```python
from build123d import *

# Parameters (mm, degrees)
BOSS_EXTRUDE1_DEPTH     = 35
SKETCH2_R               = 1.5
CUT_EXTRUDE1_DEPTH      = 31
CUT_EXTRUDE1_DEPTH_BACK = 31
SKETCH3_R               = 1.75
CUT_EXTRUDE2_DEPTH      = 6
FILLET1_R               = 4
FILLET2_R               = 2
CHAMFER1_SIZE           = 0.5


with BuildPart() as part:
    # Sketch1 → Boss-Extrude1 (new body)
    with BuildSketch(Plane.XY):
        with BuildLine():
            ThreePointArc((-10, -15.801582199), (-18.048902858, 4.891534078), (-0.652620588, 18.688608465))
            Line((-0.652620588, 18.688608465), (-0.792218575, 22.686171773))
            ThreePointArc((-0.792218575, 22.686171773), (-2.292863817, 22.583905232), (-3.783442178, 22.382483448))
            ThreePointArc((-3.783442178, 22.382483448), (-22.463854977, 3.265764775), (-10, -20.378665314))
            Line((-10, -20.378665314), (-10, -15.801582199))
        make_face()
        with BuildLine():
            Line((0, -22.7), (0, -18.7))
            ThreePointArc((0, -18.7), (-5.205785862, -17.960784882), (-10, -15.801582199))
            Line((-10, -15.801582199), (-10, -20.378665314))
            ThreePointArc((-10, -20.378665314), (-5.132947368, -22.112052173), (0, -22.7))
        make_face()
        with BuildLine():
            ThreePointArc((10, -15.801582199), (5.205785862, -17.960784882), (0, -18.7))
            Line((0, -18.7), (0, -22.7))
            ThreePointArc((0, -22.7), (5.132947368, -22.112052173), (10, -20.378665314))
            Line((10, -20.378665314), (10, -15.801582199))
        make_face()
        with BuildLine():
            Line((0.792218575, 22.686171773), (0.652620588, 18.688608465))
            ThreePointArc((0.652620588, 18.688608465), (18.048902858, 4.891534078), (10, -15.801582199))
            Line((10, -15.801582199), (10, -20.378665314))
            ThreePointArc((10, -20.378665314), (22.463854977, 3.265764775), (3.783442178, 22.382483448))
            ThreePointArc((3.783442178, 22.382483448), (2.292863817, 22.583905232), (0.792218575, 22.686171773))
        make_face()
        with BuildLine():
            ThreePointArc((10, -20.378665314), (5.132947368, -22.112052173), (0, -22.7))
            Line((0, -22.7), (0, -32))
            Line((0, -32), (30, -32))
            Line((30, -32), (30, -27))
            Line((30, -27), (16.621334686, -27))
            ThreePointArc((16.621334686, -27), (11.939344029, -25.060655971), (10, -20.378665314))
        make_face()
        with BuildLine():
            Line((0, -32), (0, -22.7))
            ThreePointArc((0, -22.7), (-5.132947368, -22.112052173), (-10, -20.378665314))
            ThreePointArc((-10, -20.378665314), (-11.939344029, -25.060655971), (-16.621334686, -27))
            Line((-16.621334686, -27), (-30, -27))
            Line((-30, -27), (-30, -32))
            Line((-30, -32), (0, -32))
        make_face()
        with BuildLine():
            ThreePointArc((-3.783442178, 22.382483448), (-2.292863817, 22.583905232), (-0.792218575, 22.686171773))
            Line((-0.792218575, 22.686171773), (-1.029566174, 29.482917727))
            Line((-1.029566174, 29.482917727), (-4.027738655, 29.378219237))
            Line((-4.027738655, 29.378219237), (-3.783442178, 22.382483448))
        make_face()
        with BuildLine():
            Line((1.029566174, 29.482917727), (0.792218575, 22.686171773))
            ThreePointArc((0.792218575, 22.686171773), (2.292863817, 22.583905232), (3.783442178, 22.382483448))
            Line((3.783442178, 22.382483448), (4.027738655, 29.378219237))
            Line((4.027738655, 29.378219237), (1.029566174, 29.482917727))
        make_face()
    extrude(amount=BOSS_EXTRUDE1_DEPTH)

    # Sketch2 → Cut-Extrude1 (cut, two sides)
    with BuildSketch(Plane(origin=(0, 0, 0), x_dir=(0, 0, -1), z_dir=(1, 0, 0))) as cut_extrude1_sk:
        with Locations((-30, 25.880351342)):
            Circle(SKETCH2_R)
        with Locations((-5, 25.880351342)):
            Circle(SKETCH2_R)
    extrude(amount=CUT_EXTRUDE1_DEPTH, mode=Mode.SUBTRACT)
    extrude(cut_extrude1_sk.sketch, amount=-CUT_EXTRUDE1_DEPTH_BACK, mode=Mode.SUBTRACT)

    # Sketch3 → Cut-Extrude2 (cut, through all)
    with BuildSketch(Plane(origin=(0, -27, 0), x_dir=(1, 0, 0), z_dir=(0, 1, 0))):
        with Locations((-25, -5)):
            Circle(SKETCH3_R)
        with Locations((-25, -30)):
            Circle(SKETCH3_R)
        with Locations((25, -30)):
            Circle(SKETCH3_R)
        with Locations((25, -5)):
            Circle(SKETCH3_R)
    extrude(amount=-CUT_EXTRUDE2_DEPTH, mode=Mode.SUBTRACT)

    # Fillet1
    fillet1_edges = [part.edges().sort_by_distance(p)[0] for p in [
        (-10, -20.378665314, 17.5),
        (10, -20.378665314, 17.5),
    ]]
    fillet(fillet1_edges, radius=FILLET1_R)

    # Fillet2
    fillet2_edges = [part.edges().sort_by_distance(p)[0] for p in [
        (-3.783442178, 22.382483448, 17.5),
        (-0.652620588, 18.688608465, 17.5),
        (0.652620588, 18.688608465, 17.5),
        (3.783442178, 22.382483448, 17.5),
    ]]
    fillet(fillet2_edges, radius=FILLET2_R)

    # Chamfer1
    chamfer1_edges = [part.edges().sort_by_distance(p)[0] for p in [
        (30, -29.5, 35),
        (-0.874302959, 25.03676097, 0),
        (-0.874302959, 25.03676097, 35),
        (-22.357902089, 3.926094008, 0),
        (-17.579381492, -6.376154512, 0),
        (0.874302959, 25.03676097, 0),
        (1.190855047, 19.229149784, 0),
        (-1.190855047, 19.229149784, 0),
        (-17.579381492, -6.376154512, 35),
        (0.874302959, 25.03676097, 35),
        (-22.357902089, 3.926094008, 35),
        (1.190855047, 19.229149784, 35),
        (-1.190855047, 19.229149784, 35),
        (4.247231716, 22.791302098, 0),
        (4.247231716, 22.791302098, 35),
        (-4.247231716, 22.791302098, 0),
        (-4.247231716, 22.791302098, 35),
        (23.310667343, -27, 35),
        (-30, -29.5, 0),
        (-23.310667343, -27, 0),
        (-14.099306205, -26.500874504, 0),
        (-3.935041139, 26.723709689, 0),
        (-2.528652414, 29.430568482, 0),
        (14.099306205, -26.500874504, 35),
        (2.528652414, 29.430568482, 0),
        (3.935041139, 26.723709689, 0),
        (14.099306205, -26.500874504, 0),
        (23.310667343, -27, 0),
        (30, -29.5, 0),
        (0, -32, 0),
        (3.935041139, 26.723709689, 35),
        (-30, -32, 17.5),
        (-30, -27, 17.5),
        (30, -27, 17.5),
        (30, -32, 17.5),
        (2.528652414, 29.430568482, 35),
        (0, -32, 35),
        (-2.528652414, 29.430568482, 35),
        (-3.935041139, 26.723709689, 35),
        (-14.099306205, -26.500874504, 35),
        (-23.310667343, -27, 35),
        (-30, -29.5, 35),
        (22.357902089, 3.926094008, 0),
        (22.357902089, 3.926094008, 35),
        (-10.793982585, -21.849764719, 0),
        (-10.793982585, -21.849764719, 35),
        (10.793982585, -21.849764719, 0),
        (10.793982585, -21.849764719, 35),
    ]]
    chamfer(chamfer1_edges, length=CHAMFER1_SIZE)


solid = part.part
```
Source: CAD feature listing. Evaluate the final solid. Frame: model axes, mm. A direction names the side the tool comes from. Round coordinates to 2 decimals unless told otherwise and drop trailing zeros. Loops run counter-clockwise (first coordinate to the right, second up) from the corner with the lowest first, then second, coordinate; pieces in that order, holes last. Notation, with made-up numbers: (58.5, 45) - (97.5, 45) arc R30 cw to (97.5, 82) - close; hole circle Ø3 at (-15, 79). An arc over 180 degrees is marked (long way). Use CSV: the item, a comma, the result in double quotes.
Q1. Ray query, line 1 along X through (y, z) = (-30.05, 5); line 2 along X through (y, z) = (24, 24.5); line 3 along Y through (x, z) = (12, 8). Return the intervals inside material, ascending.
Reported:
line 1,"-30 to -26.75, -23.25 to 23.25, 26.75 to 30"
line 2,"-3.84 to -0.84, 0.84 to 3.84"
line 3,"-32 to -25.12, -19.36 to -14.34, 14.34 to 19.27"
Q2. Pin query (flat end, axial travel): pin 1 Ø3 at (y, z) = (-7.5, 27.5) entering from +X; pin 2 Ø14 at (x, z) = (-26, 14) entering from +Y; pin 3 Ø14 at (x, z) = (24.5, 12.5) entering from +Y. Return the tip coordinate at first contact, or that it passes through.
Reported:
pin 1,"x = 21.89"
pin 2,"y = 12.42"
pin 3,"y = 14.46"
Q3. Reachability of faces 1 (the cylindrical face through (4.259, 22.776, 17.738)), 2 (the conical face through (-14.011, -26.618, 34.642)), 3 (the conical face through (14.079, -26.647, 34.642)), 4 (the cylindrical face through (1.204, 19.213, 17.738)) from +Z, -Z, +X, -X, +Y, -Y: full face, straight path, thin tool, end or side. Return the list, or none.
Reported:
face 1,"+Z, -Z, +X"
face 2,"+Z, -X"
face 3,"+Z, +X"
face 4,"+Z, -Z"
Q4. Section query B-B, the plane z = 5. Give the number of separate pieces and of enclosed holes in the cut face, then the cut area to 3 significant figures.
Reported:
separate pieces,"5"
enclosed holes,"0"
area,"927 mm^2"
Q5. Mould query, pull axis Y, two halves, no side actions, for faces 5 (the flat face through (2, -21, 0)), 6 (the cylindrical face through (22.42, 3.56, 17.26)). Classes: pulls with the +Y half, pulls with the -Y half, needs draft (parallel to the pull), parting line crosses it, or undercut.
Reported:
face 5,"needs draft"
face 6,"undercut"
Q6. Section query A-A, the plane x = 25. Output: boundary loops of the cut face in (y, z).
Reported:
outline,"(-32, 0.5) - (-31.5, 0) - (-27.5, 0) - (-27, 0.5) - (-27, 3.25) - (-32, 3.25) - close; (-32, 6.75) - (-27, 6.75) - (-27, 28.25) - (-32, 28.25) - close; (-32, 31.75) - (-27, 31.75) - (-27, 34.5) - (-27.5, 35) - (-31.5, 35) - (-32, 34.5) - close"
